Work out the finished part from the listing and answer in its coordinate system (mm). A direction names the side the tool comes from. Give positions to 0.01 mm unless a question says otherwise; leave off trailing zeros. Write each loop counter-clockwise with the first axis right and the second up, starting at its lowest first coordinate (ties: lowest second). Pieces come first, ordered by that corner, then holes. Notation, with made-up numbers: (85, 25) -> (114, 25) arc R22 cw to (114, 54) -> close; hole circle Ø1 at (68.25, -19.5). An arc over 180 degrees is marked (long way). Use a Markdown table: item, result. Add a question column.
Q1. Section B-B, the plane z = 50 is taken. Give the vertices of the cut face in (x, y), plus the area to 3 significant figures.
Q2. Each of these flat-tipped pins is pushed along its axis until it touches: pin 1 Ø4.5 at (y, z) = (363, 12) entering from +X; pin 2 Ø4 at (x, y) = (94.5, 167.5) entering from +Z; pin 3 Ø5 at (x, z) = (93.5, 17.5) entering from +Y. Where does it stop, or does it pass through?
Q3. Section C-C, the plane y = 80 is taken. Give the vertices of the cut face in (x, z).
Q4. Section A-A, the plane x = 185 is taken. Give the vertices of the cut face in (y, z).
Q5. For faces 1 (the face through (-100, 536, 214)), 2 (the face through (87, 33, 15)), 3 (the face through (117, 361, 12)), 4 (the face through (37, 361, 12)), 5 (the face through (-98, 234, 15)), determine the directions among +Z, -Z, +X, -X, +Y, -Y from which every point of the face is accessible in a straight line to the end or side of a thin tool.
Q6. Section D-D, the plane y = 436 is taken. Give the vertices of the cut face in (x, z).
Q7. For a pull along Y with two mould halves and no side action, classify faces 6 (the face through (-3, 0, 128)), 7 (the face through (107, 290, 17)), 8 (the face through (-88, 107, 15)) as pulls with the +Y half, pulls with the -Y half, needs draft (parallel to the pull), parting line crosses it, or undercut.
Q8. Consider line 1 (Y direction, x = 111, z = 16.5); line 2 (X direction, y = 40, z = 2); line 3 (Y direction, x = -185, z = 2). Determine where each line is inside the solid, lowest interval first.
from build123d import *

# Parameters (mm, degrees)
SKETCH1_W                  = 400
SKETCH1_H                  = 560
PANEL_DEPTH                = 5
SKETCH2_W                  = 394
SKETCH2_H                  = 255
SHELF_DEPTH                = 5
WALL_KEYHOLES_DEPTH        = 649.999229584
WALL_KEYHOLES_DEPTH_BACK   = 649.999229584
SKETCH3_W                  = 14
SKETCH3_H                  = 26
CONNECTOR_HOLES_DEPTH      = 649.999229584
CONNECTOR_HOLES_DEPTH_BACK = 649.999229584
SKETCH4_R                  = 6.2
SKETCH4_R_2                = 4.1
MODULE_POSTS_START         = 5
SKETCH5_R                  = 6
MODULE_POSTS_DEPTH         = 209
SADDLES_SED_START          = 5
SKETCH6_W                  = 16
SKETCH6_H                  = 14
SADDLES_SED_DEPTH          = 20
SADDLES_CARB_START         = 5
SKETCH7_W                  = 16
SKETCH7_H                  = 14
SADDLES_CARB_DEPTH         = 20
SADDLES_RO_START           = 5
SKETCH8_W                  = 16
SKETCH8_H                  = 14
SADDLES_RO_DEPTH           = 14
SADDLES_UF_START           = 5
SKETCH9_W                  = 16
SKETCH9_H                  = 14
SADDLES_UF_DEPTH           = 20
SADDLES_UVC_START          = 5
SKETCH10_W                 = 16
SKETCH10_H                 = 14
SADDLES_UVC_DEPTH          = 25
PUMP_MOUNT_POSTS_START     = 5
SKETCH11_W                 = 16
SKETCH11_H                 = 30
PUMP_MOUNT_POSTS_DEPTH     = 15
LABEL_IN_START             = 5
SKETCH12_W                 = 1.538461538
SKETCH12_H                 = 8
LABEL_IN_DEPTH             = 0.6


with BuildPart() as part:
    # Sketch1 → Panel (new body)
    with BuildSketch(Plane.XY):
        with Locations((0, 280)):
            Rectangle(SKETCH1_W, SKETCH1_H)
    extrude(amount=PANEL_DEPTH)

    # Sketch2 → Shelf (add)
    with BuildSketch(Plane(origin=(0, 0, 0), x_dir=(1, 0, 0), z_dir=(0, 1, 0))):
        with Locations((0, -132.5)):
            Rectangle(SKETCH2_W, SKETCH2_H)
    extrude(amount=SHELF_DEPTH)

    # Sketch3 → Wall_Keyholes (cut, two sides: drawn at the far end of the back side and taken through both)
    with BuildSketch(Plane.XY.offset(-WALL_KEYHOLES_DEPTH_BACK)):
        with Locations((-120, 520)):
            Rectangle(SKETCH3_W, SKETCH3_H)
        with Locations((120, 520)):
            Rectangle(SKETCH3_W, SKETCH3_H)
    extrude(amount=WALL_KEYHOLES_DEPTH + WALL_KEYHOLES_DEPTH_BACK, mode=Mode.SUBTRACT)

    # Sketch4 → Connector_Holes (cut, two sides: drawn at the far end of the back side and taken through both)
    with BuildSketch(Plane.XY.offset(-CONNECTOR_HOLES_DEPTH_BACK)):
        with Locations((-185, 40)):
            Circle(SKETCH4_R)
        with Locations((185, 80)):
            Circle(SKETCH4_R)
        with Locations((-150, 480)):
            Circle(SKETCH4_R_2)
    extrude(amount=CONNECTOR_HOLES_DEPTH + CONNECTOR_HOLES_DEPTH_BACK, mode=Mode.SUBTRACT)

    # Sketch5 → Module_Posts (add)
    with BuildSketch(Plane.XY.offset(MODULE_POSTS_START)):
        with Locations((-100, 436)):
            Circle(SKETCH5_R)
        with Locations((-100, 536)):
            Circle(SKETCH5_R)
        with Locations((100, 436)):
            Circle(SKETCH5_R)
        with Locations((100, 536)):
            Circle(SKETCH5_R)
    extrude(amount=MODULE_POSTS_DEPTH)

    # Sketch6 → Saddles_SED (add)
    with BuildSketch(Plane.XY.offset(SADDLES_SED_START)):
        with Locations((-87.5, 40)):
            Rectangle(SKETCH6_W, SKETCH6_H)
        with Locations((87.5, 40)):
            Rectangle(SKETCH6_W, SKETCH6_H)
    extrude(amount=SADDLES_SED_DEPTH)

    # Sketch7 → Saddles_CARB (add)
    with BuildSketch(Plane.XY.offset(SADDLES_CARB_START)):
        with Locations((-87.5, 100)):
            Rectangle(SKETCH7_W, SKETCH7_H)
        with Locations((87.5, 100)):
            Rectangle(SKETCH7_W, SKETCH7_H)
    extrude(amount=SADDLES_CARB_DEPTH)

    # Sketch8 → Saddles_RO (add)
    with BuildSketch(Plane.XY.offset(SADDLES_RO_START)):
        with Locations((-110, 167)):
            Rectangle(SKETCH8_W, SKETCH8_H)
        with Locations((110, 167)):
            Rectangle(SKETCH8_W, SKETCH8_H)
    extrude(amount=SADDLES_RO_DEPTH)

    # Sketch9 → Saddles_UF (add)
    with BuildSketch(Plane.XY.offset(SADDLES_UF_START)):
        with Locations((-90, 234)):
            Rectangle(SKETCH9_W, SKETCH9_H)
        with Locations((90, 234)):
            Rectangle(SKETCH9_W, SKETCH9_H)
    extrude(amount=SADDLES_UF_DEPTH)

    # Sketch10 → Saddles_UVC (add)
    with BuildSketch(Plane.XY.offset(SADDLES_UVC_START)):
        with Locations((-105, 290)):
            Rectangle(SKETCH10_W, SKETCH10_H)
        with Locations((115, 290)):
            Rectangle(SKETCH10_W, SKETCH10_H)
    extrude(amount=SADDLES_UVC_DEPTH)

    # Sketch11 → Pump_Mount_Posts (add)
    with BuildSketch(Plane.XY.offset(PUMP_MOUNT_POSTS_START)):
        with Locations((45, 361)):
            Rectangle(SKETCH11_W, SKETCH11_H)
        with Locations((125, 361)):
            Rectangle(SKETCH11_W, SKETCH11_H)
    extrude(amount=PUMP_MOUNT_POSTS_DEPTH)

    # Sketch12 → Label_IN (add)
    with BuildSketch(Plane.XY.offset(LABEL_IN_START)):
        with Locations((-58.512820513, 24)):
            Rectangle(SKETCH12_W, SKETCH12_H)
        Polygon((-56.102564103, 20), (-56.102564103, 28), (-54.495192308, 28), (-51.282051282, 22.740384615), (-51.282051282, 28), (-49.743589744, 28), (-49.743589744, 20), (-51.400641026, 20), (-54.564102564, 25.176282051), (-54.564102564, 20), align=None)
    extrude(amount=LABEL_IN_DEPTH)


solid = part.part
Result set:
| question | item | result |
|---|---|---|
| 1 | outline | (-197, 0) -> (197, 0) -> (197, 5) -> (-197, 5) -> close; circle Ø12 at (-100, 436); circle Ø12 at (-100, 536); circle Ø12 at (100, 436); circle Ø12 at (100, 536) |
| 1 | area | 2,420 mm2 |
| 2 | pin 1 | stops at x = 133 |
| 2 | pin 2 | stops at z = 5 |
| 2 | pin 3 | stops at y = 540.47 |
| 3 | outline | (-200, 0) -> (178.8, 0) -> (178.8, 5) -> (-200, 5) -> close; (191.2, 0) -> (200, 0) -> (200, 5) -> (191.2, 5) -> close |
| 4 | outline | (0, 0) -> (73.8, 0) -> (73.8, 5) -> (5, 5) -> (5, 260) -> (0, 260) -> close; (86.2, 0) -> (560, 0) -> (560, 5) -> (86.2, 5) -> close |
| 5 | face 1 | +Z, +X, -X, +Y |
| 5 | face 2 | +Z, +X, -X |
| 5 | face 3 | +Z, +Y |
| 5 | face 4 | +Z, -X, +Y |
| 5 | face 5 | +Z, -X |
| 6 | outline | (-200, 0) -> (200, 0) -> (200, 5) -> (106, 5) -> (106, 214) -> (94, 214) -> (94, 5) -> (-94, 5) -> (-94, 214) -> (-106, 214) -> (-106, 5) -> (-200, 5) -> close |
| 7 | face 6 | pulls with the -Y half |
| 7 | face 7 | needs draft |
| 7 | face 8 | undercut |
| 8 | line 1 | y = 0 to 5, 160 to 174, 283 to 297 |
| 8 | line 2 | x = -200 to -191.2, -178.8 to 200 |
| 8 | line 3 | y = 0 to 33.8, 46.2 to 560 |
